from build123d import *

# Parameters (mm, degrees)
SKETCH1_R           = 3
BOSS_EXTRUDE1_DEPTH = 3
SKETCH2_W           = 32.6
SKETCH2_H           = 9.75
CUT_EXTRUDE1_DEPTH  = 2.2
CHAMFER1_SIZE       = 1
CHAMFER3_SIZE       = 0.5


with BuildPart() as part:
    # Sketch1 → Boss-Extrude1 (new body)
    with BuildSketch(Plane(origin=(0, 0, 0), x_dir=(0, 1, 0), z_dir=(0, 0, 1))):
        with BuildLine():
            Line((-25, 26), (25, 26))
            ThreePointArc((25, 26), (25.707106781, 25.707106781), (26, 25))
            Line((26, 25), (26, 6.375))
            Line((26, 6.375), (26, -6.375))
            Line((26, -6.375), (26, -25))
            ThreePointArc((26, -25), (25.707106781, -25.707106781), (25, -26))
            Line((25, -26), (-25, -26))
            ThreePointArc((-25, -26), (-25.707106781, -25.707106781), (-26, -25))
            Line((-26, -25), (-26, -6.375))
            Line((-26, -6.375), (-26, 6.375))
            Line((-26, 6.375), (-26, 25))
            ThreePointArc((-26, 25), (-25.707106781, 25.707106781), (-25, 26))
        make_face()
        with Locations(Location((-20, 20, 0), (0, 0, 270))):
            Circle(SKETCH1_R, mode=Mode.SUBTRACT)
        with Locations(Location((20, 20, 0), (0, 0, 270))):
            Circle(SKETCH1_R, mode=Mode.SUBTRACT)
        with Locations(Location((20, -20, 0), (0, 0, 270))):
            Circle(SKETCH1_R, mode=Mode.SUBTRACT)
        with Locations(Location((-20, -20, 0), (0, 0, 270))):
            Circle(SKETCH1_R, mode=Mode.SUBTRACT)
        with BuildLine():
            Line((-2.46, 18.05), (2.46, 18.05))
            ThreePointArc((2.46, 18.05), (3.697436867, 17.537436867), (4.21, 16.3))
            Line((4.21, 16.3), (4.21, -16.3))
            ThreePointArc((4.21, -16.3), (3.697436867, -17.537436867), (2.46, -18.05))
            Line((2.46, -18.05), (-2.46, -18.05))
            ThreePointArc((-2.46, -18.05), (-3.697436867, -17.537436867), (-4.21, -16.3))
            Line((-4.21, -16.3), (-4.21, 16.3))
            ThreePointArc((-4.21, 16.3), (-3.697436867, 17.537436867), (-2.46, 18.05))
        make_face(mode=Mode.SUBTRACT)
    extrude(amount=BOSS_EXTRUDE1_DEPTH)

    # Sketch2 → Cut-Extrude1 (cut)
    with BuildSketch(Plane(origin=(0, 0, 0), x_dir=(1, 0, 0), z_dir=(0, 0, -1))):
        Rectangle(SKETCH2_W, SKETCH2_H)
    extrude(amount=-CUT_EXTRUDE1_DEPTH, mode=Mode.SUBTRACT)

    # Chamfer1
    chamfer1_edges = [part.edges().sort_by_distance(p)[0] for p in [
        (17.537436867, -3.697436867, 0),
        (18.05, 0, 0),
        (17.537436867, 3.697436867, 0),
        (-17.537436867, 3.697436867, 0),
        (-18.05, 0, 0),
        (-17.537436867, -3.697436867, 0),
        (16.3, 4.5425, 0),
        (-16.3, 4.5425, 0),
        (0, 4.875, 0),
        (-16.3, -4.5425, 0),
        (16.3, -4.5425, 0),
        (0, -4.875, 0),
    ]]
    chamfer(chamfer1_edges, length=CHAMFER1_SIZE)

    # Chamfer3
    chamfer3_edges = [part.edges().sort_by_distance(p)[0] for p in [
        (25.707106781, -25.707106781, 3),
        (26, 0, 3),
        (25.707106781, 25.707106781, 3),
        (0, 26, 3),
        (-23, -20, 3),
        (-23, 20, 3),
        (17, 20, 3),
        (-25.707106781, 25.707106781, 3),
        (17, -20, 3),
        (-26, 0, 3),
        (-25.707106781, -25.707106781, 3),
        (17.537436867, -3.697436867, 3),
        (18.05, 0, 3),
        (17.537436867, 3.697436867, 3),
        (0, 4.21, 3),
        (-17.537436867, 3.697436867, 3),
        (-18.05, 0, 3),
        (-17.537436867, -3.697436867, 3),
        (0, -4.21, 3),
        (0, -26, 3),
    ]]
    chamfer(chamfer3_edges, length=CHAMFER3_SIZE)


solid = part.part
The listing builds one solid part. Answer for the finished solid, in the listing's coordinates (mm). A direction names the side the tool comes from. Round coordinates to 2 decimals unless told otherwise and drop trailing zeros. Write each loop counter-clockwise with the first axis right and the second up, starting at its lowest first coordinate (ties: lowest second). Pieces come first, ordered by that corner, then holes. Notation, with made-up numbers: M -18,34.5 L -3,34.5 A21 ccw -3,72.5 Z; hole C 29,58 d8. An arc over 180 degrees is marked long. Write each question's results on one line, items separated by ' | '. Start each with the question number.
(1) Find the intervals of material crossed by line 1 (Y direction, x = 20, z = 1.85); line 2 (Y direction, x = -7.5, z = 2) (3 decimals); line 3 (X direction, y = -4.5, z = 2.15), in increasing order.
(2) For faces 1 (the flat face through (0, -4.875, 2)), 2 (the conical face through (-17.62, -3.81, 2.64)), 3 (the flat face through (0, 26, 1)), 4 (the flat face through (-18.05, 0, 2)), determine the directions among +Z, -Z, +X, -X, +Y, -Y from which every point of the face is accessible in a straight line to the end or side of a thin tool.
(3) Determine the mould class of faces 5 (the flat face through (-0.4, 6.1, 0)), 6 (the cylindrical face through (-22.4, -21.8, 1.2)), 7 (the flat face through (26, 0, 1)) for opening direction X: +X half, -X half, draft (parallel to the pull), parting line (faces both ways), or undercut.
(4) The part is cut by section C-C, the plane x = -20. Write down the section's boundary in (y, z).
(5) This flat-tipped pin is pushed along its axis until it touches: P1, Ø0.5, axis at x = 5.5, y = -4.5, coming from the -Z side. Where does it stop, or does it pass through?
(6) The part is cut by section A-A, the plane z = 1.6. Write down the section's boundary in (x, y) (3 decimals).
(7) The part is cut by section B-B, the plane y = 1.5. Write down the section's boundary in (x, z).
Worked answers:
1) line 1: y = -26 to -23, -17 to 17, 23 to 26 | line 2: y = -26 to -4.875, 4.875 to 26 | line 3: x = -26 to -16.3, 16.3 to 26
2) face 1: -Z | face 2: +Z | face 3: +Z, -Z, +X, -X, +Y | face 4: +Z, -Z
3) face 5: draft | face 6: undercut | face 7: +X half
4) outline: M -26,0 L -23,0 L -23,2.5 L -23.5,3 L -25.5,3 L -26,2.5 Z; M -17,0 L 17,0 L 17,2.5 L 16.5,3 L -16.5,3 L -17,2.5 Z; M 23,0 L 26,0 L 26,2.5 L 25.5,3 L 23.5,3 L 23,2.5 Z
5) P1: stops at z = 2.2
6) outline: M -26,-25 A1 ccw -25,-26 L 25,-26 A1 ccw 26,-25 L 26,25 A1 ccw 25,26 L -25,26 A1 ccw -26,25 Z; hole C -20,-20 d6; hole C -20,20 d6; hole M -18.05,-2.46 A1.75 ccw -16.3,-4.21 L -16.3,-4.875 L 16.3,-4.875 L 16.3,-4.21 A1.75 ccw 18.05,-2.46 L 18.05,2.46 A1.75 ccw 16.3,4.21 L 16.3,4.875 L -16.3,4.875 L -16.3,4.21 A1.75 ccw -18.05,2.46 Z; hole C 20,-20 d6; hole C 20,20 d6
7) outline: M -26,0 L -19.05,0 L -18.05,1 L -18.05,2.5 L -18.55,3 L -25.5,3 L -26,2.5 Z; M 18.05,1 L 19.05,0 L 26,0 L 26,2.5 L 25.5,3 L 18.55,3 L 18.05,2.5 Z
